Work out the finished part from the listing and answer in its coordinate system (mm). A direction names the side the tool comes from. Coordinates: 2 decimals unless noted, no trailing zeros. Loops run counter-clockwise (first coordinate to the right, second up) from the corner with the lowest first, then second, coordinate; pieces in that order, holes last. Notation, with made-up numbers: (-6.5, 76) - (38.5, 76) arc R25 cw to (38.5, 97) - close; hole circle Ø4 at (58.25, 25.5). An arc over 180 degrees is marked (long way). Write each question's results on one line, items separated by ' | '. Start each with the question number.
Item 1: Section D-D, the plane z = 16 is taken. Write down the section's boundary in (x, y).
Item 2: Section B-B, the plane z = 0 is taken. Write down the section's boundary in (x, y), plus the area to 3 significant figures.
Item 3: For a pull along Z with two mould halves and no side action, classify faces 1 (the face through (0, 1, 19.05)), 2 (the face through (0, 0, 12)), 3 (the face through (0, -1.2, 18)) as +Z half, -Z half, draft (parallel to the pull), parting line (faces both ways), or undercut.
Item 4: Each of these flat-tipped pins is pushed along its axis until it touches: pin 1 Ø1 at (y, z) = (-2, 0.5) entering from +X; pin 2 Ø0.8 at (x, z) = (-1.5, -3) entering from +Y; pin 3 Ø1.9 at (x, z) = (5.5, 18.5) entering from -Y; pin 4 Ø1 at (y, z) = (12.5, 11) entering from +X. Where does it stop, or does it pass through?
Item 5: Section C-C, the plane z = -11 is taken. Write down the section's boundary in (x, y).
Item 6: A tool of negligible diameter and unlimited length cuts with its end or side. For faces 4 (the face through (0, -2, 7.5)), 5 (the face through (-11.43, 3, -5)), 6 (the face through (7.5, -2, 0)), 7 (the face through (0, 9, -15.24)), 8 (the face through (-7.5, -2, 0)), from which of +Z, -Z, +X, -X, +Y, -Y can it reach the whole face along a straight path? Write none if from no direction.
Item 7: Consider probe 1 along Z at (x, y) = (-5.75, 14.9); probe 2 along Y at (x, z) = (7, -15.5); probe 3 along Y at (x, z) = (4.25, 0). Determine where each line is inside the solid, lowest interval first. Write a range as [from, to].
Item 8: Section A-A, the plane y = 21 is taken. Write down the section's boundary in (x, z).
from build123d import *

# Parameters (mm, degrees)
SKETCH1_W           = 22.86
SKETCH1_H           = 38.1
BOSS_EXTRUDE1_DEPTH = 2.4
SKETCH2_W           = 22.86
SKETCH2_H           = 15
SKETCH2_H_2         = 2.4
BOSS_EXTRUDE2_DEPTH = 1.2
SKETCH3_W           = 15
SKETCH3_H           = 15
BOSS_EXTRUDE3_DEPTH = 2
SKETCH4_W           = 22.86
SKETCH4_H           = 30.48
BOSS_EXTRUDE4_DEPTH = 22.86
SKETCH5_R           = 11.938
CUT_EXTRUDE1_DEPTH  = 40.032674774
CUT_EXTRUDE2_DEPTH  = 40.032674774
FILLET1_R           = 5
FILLET2_R           = 1
BOSS_EXTRUDE5_DEPTH = 1.2


with BuildPart() as part:
    # Sketch1 → Boss-Extrude1 (new body)
    with BuildSketch(Plane(origin=(0, 0, 0), x_dir=(1, 0, 0), z_dir=(0, 1, 0))):
        Rectangle(SKETCH1_W, SKETCH1_H)
    extrude(amount=BOSS_EXTRUDE1_DEPTH)

    # Sketch2 → Boss-Extrude2 (add)
    with BuildSketch(Plane.XZ):
        Rectangle(SKETCH2_W, SKETCH2_H)
        with Locations((0, -17.85)):
            Rectangle(SKETCH2_W, SKETCH2_H_2)
        with Locations((0, 17.85)):
            Rectangle(SKETCH2_W, SKETCH2_H_2)
    extrude(amount=BOSS_EXTRUDE2_DEPTH)

    # Sketch3 → Boss-Extrude3 (add)
    with BuildSketch(Plane.XZ.offset(1.2)):
        Rectangle(SKETCH3_W, SKETCH3_H)
    extrude(amount=BOSS_EXTRUDE3_DEPTH)

    # Sketch4 → Boss-Extrude4 (add)
    with BuildSketch(Plane(origin=(0, 2.4, 0), x_dir=(1, 0, 0), z_dir=(0, 1, 0))):
        Rectangle(SKETCH4_W, SKETCH4_H)
    extrude(amount=BOSS_EXTRUDE4_DEPTH)

    # Sketch5 → Cut-Extrude1 (cut, through all)
    with BuildSketch(Plane(origin=(11.43, 0, 0), x_dir=(0, 0, -1), z_dir=(1, 0, 0))):
        with Locations((0, 14.9)):
            Circle(SKETCH5_R)
    extrude(amount=-CUT_EXTRUDE1_DEPTH, mode=Mode.SUBTRACT)

    # Sketch6 → Cut-Extrude2 (cut, through all)
    with BuildSketch(Plane(origin=(11.43, 0, 0), x_dir=(0, 0, -1), z_dir=(1, 0, 0))):
        with BuildLine():
            Line((-15.24, 25.26), (-11.177119486, 25.26))
            ThreePointArc((-11.177119486, 25.26), (-14.187968511, 20.464094672), (-15.24, 14.9))
            Line((-15.24, 14.9), (-15.24, 25.26))
        make_face()
        with BuildLine():
            Line((15.24, 14.9), (15.24, 25.26))
            Line((15.24, 25.26), (11.177119486, 25.26))
            ThreePointArc((11.177119486, 25.26), (14.187968511, 20.464094672), (15.24, 14.9))
        make_face()
    extrude(amount=-CUT_EXTRUDE2_DEPTH, mode=Mode.SUBTRACT)

    # Fillet1
    fillet1_edges = [part.edges().sort_by_distance(p)[0] for p in [
        (0, 25.26, -11.177119486),
        (0, 25.26, 11.177119486),
    ]]
    fillet(fillet1_edges, radius=FILLET1_R)

    # Fillet2
    fillet2_edges = [part.edges().sort_by_distance(p)[0] for p in [
        (0, 25.26, 5.93179939),
        (0, 25.26, -5.93179939),
    ]]
    fillet(fillet2_edges, radius=FILLET2_R)

    # Sketch7 → Boss-Extrude5 (add)
    with BuildSketch(Plane(origin=(0, 2.4, 0), x_dir=(1, 0, 0), z_dir=(0, 1, 0))):
        Polygon((-4.57, 2.2), (1.43, 2.2), (1.43, 4.6), align=None)
        Polygon((1.43, -4.6), (-4.57, -2.2), (1.43, -2.2), align=None)
    extrude(amount=BOSS_EXTRUDE5_DEPTH)


solid = part.part
Answer key:
1) outline: (-11.43, 0) - (11.43, 0) - (11.43, 2.4) - (-11.43, 2.4) - close
2) outline: (-11.43, -1.2) - (-7.5, -1.2) - (-7.5, -3.2) - (7.5, -3.2) - (7.5, -1.2) - (11.43, -1.2) - (11.43, 2.96) - (-11.43, 2.96) - close | area: 125 mm^2
3) face 1: +Z half | face 2: undercut | face 3: draft
4) pin 1: stops at x = 7.5 | pin 2: stops at y = 3.6 | pin 3: stops at y = -1.2 | pin 4: passes through
5) outline: (-11.43, 0) - (11.43, 0) - (11.43, 10.26) - (-11.43, 10.26) - close; (-11.43, 19.54) - (11.43, 19.54) - (11.43, 24.71) - (-11.43, 24.71) - close
6) face 4: +X, -X, -Y | face 5: +Z, -Z, -X, +Y, -Y | face 6: +Z, -Z, +X, -Y | face 7: -Z, +X, -X, +Y | face 8: +Z, -Z, -X, -Y
7) probe 1: z = [-15.24, -11.94], [11.94, 15.24] | probe 2: y = [0, 2.4] | probe 3: y = [-3.2, 2.96]
8) outline: (-11.43, -13.97) - (11.43, -13.97) - (11.43, -10.26) - (-11.43, -10.26) - close; (-11.43, 10.26) - (11.43, 10.26) - (11.43, 13.97) - (-11.43, 13.97) - close
